```python
from build123d import *

# Parameters (mm, degrees)
SKETCH1_W               = 109
SKETCH1_H               = 36
BOSS_EXTRUDE1_DEPTH     = 10
SKETCH2_W               = 36
SKETCH2_H               = 7
BOSS_EXTRUDE2_DEPTH     = 90
CUT_EXTRUDE1_DEPTH      = 150.013422214
CUT_EXTRUDE1_DEPTH_BACK = 150.013422214
SKETCH3_R               = 3.5
CUT_EXTRUDE2_DEPTH      = 150.013422214
CUT_EXTRUDE2_DEPTH_BACK = 3
SKETCH4_R               = 7
CUT_EXTRUDE3_START      = -3
SKETCH5_R               = 7
CUT_EXTRUDE3_DEPTH      = 3
FILLET1_R               = 18
SKETCH6_R               = 12.5
BOSS_EXTRUDE3_DEPTH     = 10
SKETCH15_R              = 13.75
BOSS_EXTRUDE5_DEPTH     = 4.25
SKETCH7_R               = 10.5
CUT_EXTRUDE4_DEPTH      = 125.073566887
SKETCH9_R               = 0.75
SKETCH9_W               = 22.5
SKETCH9_H               = 11.8
CUT_EXTRUDE5_DEPTH      = 107.743852282
SKETCH10_W              = 33
SKETCH10_H              = 15
CUT_EXTRUDE6_DEPTH      = 4
SKETCH11_W              = 17
SKETCH11_H              = 32
BOSS_EXTRUDE4_DEPTH     = 7
CUT_EXTRUDE7_REACH      = 153.869
SKETCH12_R              = 0.75
SKETCH12_W              = 11.8
SKETCH12_H              = 22.5
CUT_EXTRUDE8_START      = -5
CUT_EXTRUDE8_DEPTH      = 5
FILLET3_R               = 1.5
FILLET4_R               = 4
SKETCH14_W              = 1.25
SKETCH14_H              = 1
FILLET5_R               = 1


# Some blends are built 0.0001 mm under size
with BuildPart() as part:
    # Sketch1 → Boss-Extrude1 (new body)
    with BuildSketch(Plane(origin=(0, 0, 0), x_dir=(0, 1, 0), z_dir=(0, 0, 1))):
        Rectangle(SKETCH1_W, SKETCH1_H)
    extrude(amount=BOSS_EXTRUDE1_DEPTH)

    # Sketch2 → Boss-Extrude2 (add)
    with BuildSketch(Plane.XY.offset(10)):
        with Locations((0, 51)):
            Rectangle(SKETCH2_W, SKETCH2_H)
        with Locations((0, -51)):
            Rectangle(SKETCH2_W, SKETCH2_H)
    extrude(amount=BOSS_EXTRUDE2_DEPTH)

    # Sketch3 → Cut-Extrude1 (cut, two sides: drawn at the far end of the back side and taken through both)
    with BuildSketch(Plane.XZ.offset(54.5).offset(-CUT_EXTRUDE1_DEPTH_BACK)):
        with Locations(Location((0, 82, 0), (0, 0, 270))):
            Circle(SKETCH3_R)
    extrude(amount=CUT_EXTRUDE1_DEPTH + CUT_EXTRUDE1_DEPTH_BACK, mode=Mode.SUBTRACT)

    # Sketch4 → Cut-Extrude2 (cut, two sides: drawn at the far end of the back side and taken through both)
    with BuildSketch(Plane.XZ.offset(54.5).offset(-CUT_EXTRUDE2_DEPTH_BACK)):
        with Locations(Location((0, 82, 0), (0, 0, 90))):
            Circle(SKETCH4_R)
    extrude(amount=CUT_EXTRUDE2_DEPTH + CUT_EXTRUDE2_DEPTH_BACK, mode=Mode.SUBTRACT)

    # Sketch5 → Cut-Extrude3 (cut)
    with BuildSketch(Plane(origin=(0, 54.5, 0), x_dir=(-1, 0, 0), z_dir=(0, 1, 0)).offset(CUT_EXTRUDE3_START)):
        with Locations(Location((0, 82, 0), (0, 0, 90))):
            Circle(SKETCH5_R)
    extrude(amount=CUT_EXTRUDE3_DEPTH, mode=Mode.SUBTRACT)

    # Fillet1
    fillet1_edges = [part.edges().sort_by_distance(p)[0] for p in [
        (18, -51, 100),
        (-18, -51, 100),
        (18, 51, 100),
        (-18, 51, 100),
    ]]
    fillet(fillet1_edges, radius=FILLET1_R - 0.0001)  # a hair under: the kernel refuses the full size

    # Sketch6 → Boss-Extrude3 (add)
    with BuildSketch(Plane(origin=(0, 0, 0), x_dir=(1, 0, 0), z_dir=(0, 0, -1))):
        with Locations(Location((0, 0, 0), (0, 0, 180))):
            Circle(SKETCH6_R)
    extrude(amount=BOSS_EXTRUDE3_DEPTH)

    # Sketch15 → Boss-Extrude5 (add)
    with BuildSketch(Plane(origin=(0, 0, 0), x_dir=(1, 0, 0), z_dir=(0, 0, -1))):
        with Locations(Location((0, 0, 0), (0, 0, 180))):
            Circle(SKETCH15_R)
    extrude(amount=BOSS_EXTRUDE5_DEPTH)

    # Sketch7 → Cut-Extrude4 (cut, through all)
    with BuildSketch(Plane(origin=(0, 0, -10), x_dir=(1, 0, 0), z_dir=(0, 0, -1))):
        with Locations(Location((0, 0, 0), (0, 0, 180))):
            Circle(SKETCH7_R)
    extrude(amount=-CUT_EXTRUDE4_DEPTH, mode=Mode.SUBTRACT)

    # Sketch9 → Cut-Extrude5 (cut, through all)
    with BuildSketch(Plane.XY.offset(10)):
        with Locations((-13.65, 34.588690348)):
            Circle(SKETCH9_R)
        with Locations((13.65, 34.588690348)):
            Circle(SKETCH9_R)
        with Locations((0, 34.588690348)):
            Rectangle(SKETCH9_W, SKETCH9_H)
    extrude(amount=-CUT_EXTRUDE5_DEPTH, mode=Mode.SUBTRACT)

    # Sketch10 → Cut-Extrude6 (cut)
    with BuildSketch(Plane.XY.offset(10)):
        with Locations((0, 34.588690348)):
            Rectangle(SKETCH10_W, SKETCH10_H)
    extrude(amount=-CUT_EXTRUDE6_DEPTH, mode=Mode.SUBTRACT)

    # Sketch11 → Boss-Extrude4 (add)
    with BuildSketch(Plane(origin=(0, 54.5, 0), x_dir=(-1, 0, 0), z_dir=(0, 1, 0))):
        with Locations((-25.895511194, 66)):
            Rectangle(SKETCH11_W, SKETCH11_H)
    extrude(amount=-BOSS_EXTRUDE4_DEPTH)

    # Sketch12 → Cut-Extrude7 (cut, up to next)
    with BuildSketch(Plane(origin=(0, 54.5, 0), x_dir=(-1, 0, 0), z_dir=(0, 1, 0)), mode=Mode.PRIVATE) as cut_extrude7_sk1:
        with Locations(Location((-25.895511194, 79.65, 0), (0, 0, 90))):
            Circle(SKETCH12_R)
    cut_extrude7_tool1 = extrude(cut_extrude7_sk1.sketch, amount=-CUT_EXTRUDE7_REACH, mode=Mode.PRIVATE) & part.part
    # Sketch12 → Cut-Extrude7 (cut, up to next)
    with BuildSketch(Plane(origin=(0, 54.5, 0), x_dir=(-1, 0, 0), z_dir=(0, 1, 0)), mode=Mode.PRIVATE) as cut_extrude7_sk2:
        with Locations((-25.895511194, 52.35)):
            Circle(SKETCH12_R)
    cut_extrude7_tool2 = extrude(cut_extrude7_sk2.sketch, amount=-CUT_EXTRUDE7_REACH, mode=Mode.PRIVATE) & part.part
    # Sketch12 → Cut-Extrude7 (cut, up to next)
    with BuildSketch(Plane(origin=(0, 54.5, 0), x_dir=(-1, 0, 0), z_dir=(0, 1, 0)), mode=Mode.PRIVATE) as cut_extrude7_sk3:
        with Locations((-25.895511194, 66)):
            Rectangle(SKETCH12_W, SKETCH12_H)
    cut_extrude7_tool3 = extrude(cut_extrude7_sk3.sketch, amount=-CUT_EXTRUDE7_REACH, mode=Mode.PRIVATE) & part.part
    add(cut_extrude7_tool1.solids().sort_by_distance((25.895511, 54.5, 79.65))[0], mode=Mode.SUBTRACT)
    add(cut_extrude7_tool2.solids().sort_by_distance((25.895511, 54.5, 52.35))[0], mode=Mode.SUBTRACT)
    add(cut_extrude7_tool3.solids().sort_by_distance((25.895511, 54.5, 66))[0], mode=Mode.SUBTRACT)

    # Sketch13 → Cut-Extrude8 (cut)
    with BuildSketch(Plane.XY.offset(10).offset(CUT_EXTRUDE8_START)):
        with BuildLine():
            Line((18, -10.5), (18, 10.5))
            Line((18, 10.5), (0, 10.5))
            ThreePointArc((0, 10.5), (10.5, 0), (0, -10.5))
            Line((0, -10.5), (18, -10.5))
        make_face()
    extrude(amount=CUT_EXTRUDE8_DEPTH, mode=Mode.SUBTRACT)

    # Fillet3
    fillet3_edges = [part.edges().sort_by_distance(p)[0] for p in [
        (-18, 0, 10),
        (18, -29, 10),
        (-7.424621202, 7.424621202, 10),
        (18, 29, 10),
        (9, -10.5, 10),
        (9, 10.5, 10),
    ]]
    fillet(fillet3_edges, radius=FILLET3_R - 0.0001)  # a hair under: the kernel refuses the full size

    # Fillet4
    # the kernel refuses this fillet: 4 mm, written as the material it adds along each edge
    with BuildSketch(Plane(origin=(16.5001, 47.5, 10), x_dir=(0, -1, 0), z_dir=(-1, 0, 0))) as fillet4_piece_1:
        with BuildLine():
            CenterArc((FILLET4_R, FILLET4_R), FILLET4_R, 180, 90)
            Line((0, FILLET4_R), (0, 0))
            Line((0, 0), (FILLET4_R, 0))
        make_face()
    extrude(amount=33.0002)
    with BuildSketch(Plane(origin=(16.5001, -47.5, 10), x_dir=(0, 1, 0), z_dir=(-1, 0, 0))) as fillet4_piece_2:
        with BuildLine():
            CenterArc((FILLET4_R, -FILLET4_R), FILLET4_R, 90, 90)
            Line((0, -FILLET4_R), (0, 0))
            Line((0, 0), (FILLET4_R, 0))
        make_face()
    extrude(amount=33.0002)
    with BuildSketch(Plane(origin=(-16.5001, -47.5, 8.5001), x_dir=(0, 0, 1), z_dir=(1, 0, 0))) as fillet4_piece_3_section:
        with BuildLine():
            CenterArc((1.4999 + FILLET4_R, -FILLET4_R), FILLET4_R, 90, 90)
            Line((1.4999 + FILLET4_R, 0), (1.4999, 0))
            Line((1.4999, 0), (1.4999, -FILLET4_R))
        make_face()
    fillet4_piece_3 = revolve(axis=Axis((-16.5001, -47.5, 8.5001), (0, -1, 0)), revolution_arc=359.64, mode=Mode.PRIVATE)
    fillet4_piece_3 = split(fillet4_piece_3, bisect_by=Plane(origin=(-18, -46.011467158, 9.644627934), z_dir=(1, 0, 0)), keep=Keep.TOP, mode=Mode.PRIVATE)
    add(fillet4_piece_3)
    with BuildSketch(Plane(origin=(-16.5001, 47.5, 8.5001), x_dir=(0, 0, 1), z_dir=(1, 0, 0))) as fillet4_piece_4_section:
        with BuildLine():
            CenterArc((1.4999 + FILLET4_R, FILLET4_R), FILLET4_R, 180, 90)
            Line((1.4999 + FILLET4_R, 0), (1.4999, 0))
            Line((1.4999, 0), (1.4999, FILLET4_R))
        make_face()
    fillet4_piece_4 = revolve(axis=Axis((-16.5001, 47.5, 8.5001), (0, -1, 0)), revolution_arc=359.64, mode=Mode.PRIVATE)
    fillet4_piece_4 = split(fillet4_piece_4, bisect_by=Plane(origin=(-18, 46.011467158, 9.644627939), z_dir=(1, 0, 0)), keep=Keep.TOP, mode=Mode.PRIVATE)
    add(fillet4_piece_4)
    with BuildSketch(Plane(origin=(16.5001, -47.5, 8.5001), x_dir=(-0.006283143965559021, 0, 0.9999802608561371), z_dir=(0.9999802608561371, 0, 0.006283143965559021))) as fillet4_piece_5_section:
        with BuildLine():
            CenterArc((-1.4999 - FILLET4_R, -FILLET4_R), FILLET4_R, 0, 90)
            Line((-1.4999 - FILLET4_R, 0), (-1.4999, 0))
            Line((-1.4999, 0), (-1.4999, -FILLET4_R))
        make_face()
    fillet4_piece_5 = revolve(axis=Axis((16.5001, -47.5, 8.5001), (0, -1, 0)), revolution_arc=359.64, mode=Mode.PRIVATE)
    fillet4_piece_5 = split(fillet4_piece_5, bisect_by=Plane(origin=(18, -46.011467161, 9.644627937), z_dir=(-1, 0, 0)), keep=Keep.TOP, mode=Mode.PRIVATE)
    add(fillet4_piece_5)
    with BuildSketch(Plane(origin=(16.5001, 47.5, 8.5001), x_dir=(-0.006283143965559021, 0, 0.9999802608561371), z_dir=(0.9999802608561371, 0, 0.006283143965559021))) as fillet4_piece_6_section:
        with BuildLine():
            CenterArc((-1.4999 - FILLET4_R, FILLET4_R), FILLET4_R, 270, 90)
            Line((-1.4999, FILLET4_R), (-1.4999, 0))
            Line((-1.4999, 0), (-1.4999 - FILLET4_R, 0))
        make_face()
    fillet4_piece_6 = revolve(axis=Axis((16.5001, 47.5, 8.5001), (0, -1, 0)), revolution_arc=359.64, mode=Mode.PRIVATE)
    fillet4_piece_6 = split(fillet4_piece_6, bisect_by=Plane(origin=(18, 46.011467202, 9.644627972), z_dir=(-1, 0, 0)), keep=Keep.TOP, mode=Mode.PRIVATE)
    add(fillet4_piece_6)
    # the kernel refuses this fillet: 4 mm, written as the material it takes off along each edge
    with BuildSketch(Plane(origin=(-28, -54.5, 0), x_dir=(0, 0, 1), z_dir=(1, 0, 0))) as fillet4_2_piece_1:
        with BuildLine():
            CenterArc((FILLET4_R, -FILLET4_R), FILLET4_R, 90, 90)
            Line((0, -FILLET4_R), (0, 0))
            Line((0, 0), (FILLET4_R, 0))
        make_face()
    extrude(amount=56, mode=Mode.SUBTRACT)
    with BuildSketch(Plane(origin=(28, 54.5, 0), x_dir=(0, -1, 0), z_dir=(-1, 0, 0))) as fillet4_2_piece_2:
        with BuildLine():
            CenterArc((FILLET4_R, FILLET4_R), FILLET4_R, 180, 90)
            Line((0, FILLET4_R), (0, 0))
            Line((0, 0), (FILLET4_R, 0))
        make_face()
    extrude(amount=56, mode=Mode.SUBTRACT)

    # Sketch14 → Cut-Revolve1 (revolve, cut)
    with BuildSketch(Plane.YZ, mode=Mode.PRIVATE) as cut_revolve1_sk:
        with Locations((-12.375, -8.75)):
            Rectangle(SKETCH14_W, SKETCH14_H)
    revolve(cut_revolve1_sk.sketch.rotate(Axis((0, 0, -10), (0, 0, 1)), 180), axis=Axis((0, 0, -10), (0, 0, 1)), mode=Mode.SUBTRACT)

    # Fillet5
    fillet5_edges = [part.edges().sort_by_distance(p)[0] for p in [
        (13.75, 0, 0),
    ]]
    fillet(fillet5_edges, radius=FILLET5_R)


solid = part.part
```
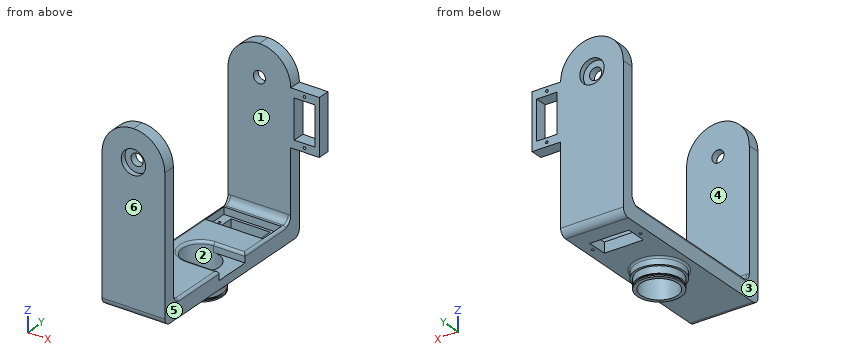
Geometry check sheet. Reference: the model listing, model coordinates, mm. Face numbers are marked on the shaded views. A direction names the side the tool comes from. Give positions to 0.01 mm unless a question says otherwise; leave off trailing zeros. Order: outer loops, then holes, each group sorted by start corner. A loop starts at its lowest first (then second) coordinate and runs counter-clockwise, first axis right, second up.
1. Access from +Z, -Z, +X, -X, +Y, -Y to the whole of each face (thin tool, end or side, straight path). Record for the marked faces 4, 5 and 6.
2. Section check B-B, the plane y = 0. Enter the section's corners in (x, z), and give its area (3 significant figures).
3. Release check for a two-part mould opening along X. For the marked faces 1, 2 and 3 record: pulls with the +X half, pulls with the -X half, needs draft (parallel to the pull), parting line crosses it, or undercut.
4. Section check A-A, the plane z = 24.5. Enter the section's corners in (x, y).
5. Section check C-C, the plane y = -18.5. Enter the section's corners in (x, z).
6. Gauge pin test, flat ends, axial feed: pin 1 Ø12.5 at (x, y) = (4.5, 3) entering from +Z; pin 2 Ø3.5 at (x, y) = (24, 51) entering from +Z; pin 3 Ø2 at (x, y) = (14, -33) entering from +Z. Record the tip position at first contact, or that the pin passes through.
7. Thickness scan on L1, parallel to Y at x = 9, z = 93; L2, parallel to X at y = 50.25, z = 52.35; L3, parallel to Z at x = 11, y = -3.5. Record the ranges inside material, lowest first.
Values follow:
1. face 4: +Z, +X, -X
1. face 5: -Z, +X, -Y
1. face 6: +Z, -Z, +X, -X, -Y
2. outline: (-18, 0) - (-14.75, 0) arc R1 cw to (-13.75, -1) - (-13.75, -4.25) - (-12.5, -4.25) - (-12.5, -8.25) - (-11.75, -8.25) - (-11.75, -9.25) - (-12.5, -9.25) - (-12.5, -10) - (-10.5, -10) - (-10.5, 8.5) arc R1.5 ccw to (-12, 10) - (-16.5, 10) arc R1.5 ccw to (-18, 8.5) - close; (10.5, -10) - (12.5, -10) - (12.5, -9.25) - (11.75, -9.25) - (11.75, -8.25) - (12.5, -8.25) - (12.5, -4.25) - (13.75, -4.25) - (13.75, -1) arc R1 cw to (14.75, 0) - (18, 0) - (18, 5) - (10.5, 5) - close
2. area: 161 mm2
3. face 1: needs draft
3. face 2: undercut
3. face 3: pulls with the -X half
4. outline: (-18, -54.5) - (18, -54.5) - (18, -47.5) - (-18, -47.5) - close; (-18, 47.5) - (18, 47.5) - (18, 54.5) - (-18, 54.5) - close
5. outline: (-18, 0) - (18, 0) - (18, 8.5) arc R1.5 ccw to (16.5, 10) - (-16.5, 10) arc R1.5 ccw to (-18, 8.5) - close
6. pin 1: stops at z = 5
6. pin 2: stops at z = 82
6. pin 3: stops at z = 10
7. L1: y = -54.5 to -47.5, 47.5 to 54.5
7. L2: x = -18 to 25.15, 26.65 to 34.4
7. L3: z = -10 to 5
